```python
from build123d import *

# Parameters (mm, degrees)
SKETCH_1_W          = 15.8
SKETCH_1_H          = 7.8
EXTRUDE_1_DEPTH     = 3.2
SKETCH_2_R          = 2.4
EXTRUDE_2_DEPTH     = 1.7
SKETCH_3_R          = 2.5
CUT_EXTRUDE_1_DEPTH = 1.8


with BuildPart() as part:
    # Эскиз1 → Бобышка-Вытянуть1 (new body)
    with BuildSketch(Plane.XY):
        Rectangle(SKETCH_1_W, SKETCH_1_H)
    extrude(amount=EXTRUDE_1_DEPTH)

    # Эскиз2 → Бобышка-Вытянуть2 (add)
    with BuildSketch(Plane(origin=(0, 0, 0), x_dir=(-1, 0, 0), z_dir=(0, 0, -1))):
        with Locations((-4, 0)):
            Circle(SKETCH_2_R)
        with Locations((4, 0)):
            Circle(SKETCH_2_R)
    extrude(amount=EXTRUDE_2_DEPTH)

    # Эскиз3 → Вырез-Вытянуть1 (cut)
    with BuildSketch(Plane.XY.offset(3.2)):
        with Locations((-4, 0)):
            Circle(SKETCH_3_R)
        with Locations((4, 0)):
            Circle(SKETCH_3_R)
    extrude(amount=-CUT_EXTRUDE_1_DEPTH, mode=Mode.SUBTRACT)


solid = part.part
```
Build history of the part. All positions in model axes, mm. A direction names the side the tool comes from. Round coordinates to 2 decimals unless told otherwise and drop trailing zeros. Write each loop counter-clockwise with the first axis right and the second up, starting at its lowest first coordinate (ties: lowest second). Pieces come first, ordered by that corner, then holes.
1) Pin check, flat tips, straight feed: pin 1 (4.5 mm diameter, centred on x = 4, y = 0, fed in from +Z); pin 2 (2.5 mm diameter, centred on x = 0, y = -1, fed in from -Z). Stop position of each tip, or through.
2) Band-saw the part on A-A, the plane z = 2.3. List the corners of the cut face in (x, y).
3) 3-axis set-ups, long thin cutter, end or side, ignore diameter. For faces 1 (the flat face through (0, 0, 3.2)), 2 (the cylindrical face through (-6.217, -0.919, -0.838)), 3 (the cylindrical face through (6.385, 0.751, 2.313)): which of +Z, -Z, +X, -X, +Y, -Y reach the whole face in a straight line?
4) Band-saw the part on B-B, the plane x = -4. List the corners of the cut face in (y, z), and give its area (3 significant figures).
5) Drill centre lines: probe 1 along Y at (x, z) = (4, 2.7); probe 2 along Z at (x, y) = (-4, -2.25); probe 3 along Z at (x, y) = (-5.25, -3). Where is each one in solid material? Low to high.
6) Band-saw the part on C-C, the plane y = 0. List the corners of the cut face in (x, z).
7) Band-saw the part on D-D, the plane x = 2. List the corners of the cut face in (y, z), and give its area (3 significant figures).
8) Mould opens along Y. For faces 4 (the flat face through (4, 0, 1.4)), 5 (the flat face through (-4, 0, 1.4)), 6 (the cylindrical face through (1.71, 0.72, -0.84)), 7 (the flat face through (-4, 0, -1.7)) say: +Y half, -Y half, draft (parallel to the pull), parting line (faces both ways), or undercut.
Ans:
1. pin 1: stops at z = 1.4
1. pin 2: stops at z = 0
2. outline: (-7.9, -3.9) - (7.9, -3.9) - (7.9, 3.9) - (-7.9, 3.9) - close; hole circle Ø5 at (-4, 0); hole circle Ø5 at (4, 0)
3. face 1: +Z, +X, -X, +Y, -Y
3. face 2: -Z
3. face 3: +Z
4. outline: (-3.9, 0) - (-2.4, 0) - (-2.4, -1.7) - (2.4, -1.7) - (2.4, 0) - (3.9, 0) - (3.9, 3.2) - (2.5, 3.2) - (2.5, 1.4) - (-2.5, 1.4) - (-2.5, 3.2) - (-3.9, 3.2) - close
4. area: 24.1 mm2
5. probe 1: y = -3.9 to -2.5, 2.5 to 3.9
5. probe 2: z = -1.7 to 1.4
5. probe 3: z = 0 to 3.2
6. outline: (-7.9, 0) - (-6.4, 0) - (-6.4, -1.7) - (-1.6, -1.7) - (-1.6, 0) - (1.6, 0) - (1.6, -1.7) - (6.4, -1.7) - (6.4, 0) - (7.9, 0) - (7.9, 3.2) - (6.5, 3.2) - (6.5, 1.4) - (1.5, 1.4) - (1.5, 3.2) - (-1.5, 3.2) - (-1.5, 1.4) - (-6.5, 1.4) - (-6.5, 3.2) - (-7.9, 3.2) - close
7. outline: (-3.9, 0) - (-1.33, 0) - (-1.33, -1.7) - (1.33, -1.7) - (1.33, 0) - (3.9, 0) - (3.9, 3.2) - (1.5, 3.2) - (1.5, 1.4) - (-1.5, 1.4) - (-1.5, 3.2) - (-3.9, 3.2) - close
7. area: 24.1 mm2
8. face 4: undercut
8. face 5: undercut
8. face 6: parting line
8. face 7: draft
